Part print with two shaded views. Sizes in mm from the minimum x, y, z corner. A direction names the side the tool comes from. Coordinates: 2 decimals unless noted, no trailing zeros. Write each loop counter-clockwise with the first axis right and the second up, starting at its lowest first coordinate (ties: lowest second). Pieces come first, ordered by that corner, then holes. Notation, with made-up numbers: (49, -4.75) - (70, -4.75) arc R8 ccw to (70, 10.25) - close; hole circle Ø9 at (-23, 79). An arc over 180 degrees is marked (long way). Answer in a Markdown table with one row per item. Add a question column.
Q1. 3-axis set-ups, long thin cutter, end or side, ignore diameter. For the marked faces 1, 2 and 3: which of +Z, -Z, +X, -X, +Y, -Y reach the whole face in a straight line?
Q2. Drill centre lines: line 1 along Z through (x, y) = (9.5, 8.75); line 2 along Z through (x, y) = (19, 1.5); line 3 along Y through (x, z) = (14, 28.5). Where is each one in solid material? Low to high. Write a range as from..to.
Q3. Pin check, flat tips, straight feed: pin 1 (4 mm diameter, centred on x = 13, z = 30.5, fed in from -Y); pin 2 (2 mm diameter, centred on x = 27.5, y = 8, fed in from +Z); pin 3 (1 mm diameter, centred on x = 15, z = 39, fed in from -Y); pin 4 (2 mm diameter, centred on x = 5.5, z = 38, fed in from -Y) (3 decimals). Stop position of each tip, or through.
Q4. Band-saw the part on C-C (x = 23.5). List the corners of the cut face in (y, z).
Q5. Band-saw the part on B-B (z = 23.9). List the corners of the cut face in (x, y).
Q6. Band-saw the part on A-A (x = 27.8). List the corners of the cut face in (y, z).
Q7. Two-plate mould, pull along Z, no slides. Class the marked faces 4, 5, 6 and 7: +Z half, -Z half, draft (parallel to the pull), parting line (faces both ways), or undercut.
Q8. Band-saw the part on D-D (z = 47.5). List the corners of the cut face in (x, y), and give its area (3 significant figures).
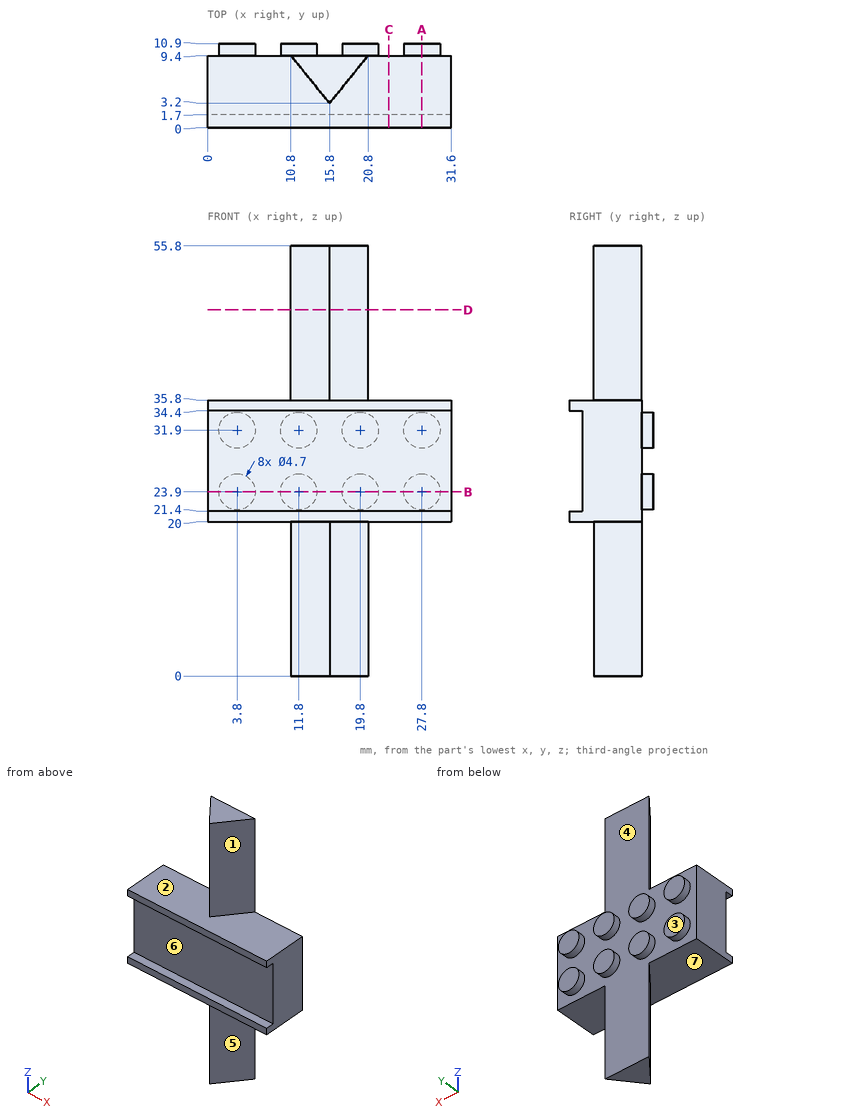
Checked values:
| question | item | result |
|---|---|---|
| 1 | face 1 | +Z, +X, -Y |
| 1 | face 2 | +Z, -Y |
| 1 | face 3 | +Z, -Z, +X, -X, +Y |
| 2 | line 1 | z = 20..35.8 |
| 2 | line 2 | z = 20..21.4, 34.4..35.8 |
| 2 | line 3 | y = 1.7..9.4 |
| 3 | pin 1 | stops at y = 1.7 |
| 3 | pin 2 | stops at z = 35.8 |
| 3 | pin 3 | stops at y = 3.57 |
| 3 | pin 4 | passes through |
| 4 | outline | (0, 20) - (9.4, 20) - (9.4, 35.8) - (0, 35.8) - (0, 34.4) - (1.7, 34.4) - (1.7, 21.4) - (0, 21.4) - close |
| 5 | outline | (0, 1.7) - (31.6, 1.7) - (31.6, 9.4) - (30.15, 9.4) - (30.15, 10.9) - (25.45, 10.9) - (25.45, 9.4) - (22.15, 9.4) - (22.15, 10.9) - (17.45, 10.9) - (17.45, 9.4) - (14.15, 9.4) - (14.15, 10.9) - (9.45, 10.9) - (9.45, 9.4) - (6.15, 9.4) - (6.15, 10.9) - (1.45, 10.9) - (1.45, 9.4) - (0, 9.4) - close |
| 6 | outline | (0, 20) - (9.4, 20) - (9.4, 21.55) - (10.9, 21.55) - (10.9, 26.25) - (9.4, 26.25) - (9.4, 29.55) - (10.9, 29.55) - (10.9, 34.25) - (9.4, 34.25) - (9.4, 35.8) - (0, 35.8) - (0, 34.4) - (1.7, 34.4) - (1.7, 21.4) - (0, 21.4) - close |
| 7 | face 4 | undercut |
| 7 | face 5 | draft |
| 7 | face 6 | undercut |
| 7 | face 7 | -Z half |
| 8 | outline | (10.8, 9.4) - (15.8, 3.2) - (20.8, 9.4) - close |
| 8 | area | 31.0 mm² |
